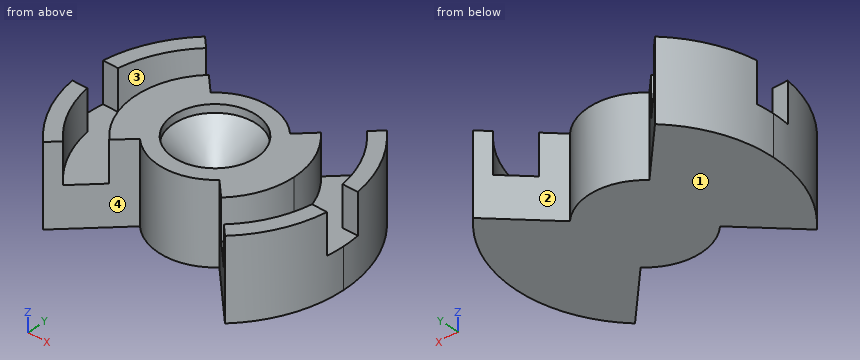
```python
from build123d import *

# Parameters (mm, degrees)
F0_R     = 3.27025
F1_DEPTH = 6.35
F2_R     = 3.27025
F3_DEPTH = 3.175
F4_SIZE  = 2.54


# Not quite as in the source:
# - a feature names something its author has since deleted; it is built from what else it names


with BuildPart() as f1:
    # F0 (on Top) → F1 (new body)
    with BuildSketch(Plane.XY):
        with BuildLine():
            ThreePointArc((-4.445, 0), (-4.106644522, 1.7010278569), (-3.1430896424, 3.1430896424))
            Line((-3.1430896424, 3.1430896424), (-7.1842048969, 7.1842048969))
            ThreePointArc((-7.1842048969, 7.1842048969), (-9.3866160503, 3.8880636728), (-10.16, 0))
            ThreePointArc((-10.16, 0), (-9.3866160503, -3.8880636728), (-7.1842048969, -7.1842048969))
            Line((-7.1842048969, -7.1842048969), (-3.1430896424, -3.1430896424))
            ThreePointArc((-3.1430896424, -3.1430896424), (-4.106644522, -1.7010278569), (-4.445, 0))
        make_face()
        with BuildLine():
            ThreePointArc((3.1430896424, -3.1430896424), (4.106644522, -1.7010278569), (4.445, 0))
            ThreePointArc((4.445, 0), (4.106644522, 1.7010278569), (3.1430896424, 3.1430896424))
            ThreePointArc((3.1430896424, 3.1430896424), (0, 4.445), (-3.1430896424, 3.1430896424))
            ThreePointArc((-3.1430896424, 3.1430896424), (-4.106644522, 1.7010278569), (-4.445, 0))
            ThreePointArc((-4.445, 0), (-4.106644522, -1.7010278569), (-3.1430896424, -3.1430896424))
            ThreePointArc((-3.1430896424, -3.1430896424), (0, -4.445), (3.1430896424, -3.1430896424))
        make_face()
        Circle(F0_R, mode=Mode.SUBTRACT)
        with BuildLine():
            ThreePointArc((3.1430896424, 3.1430896424), (4.106644522, 1.7010278569), (4.445, 0))
            ThreePointArc((4.445, 0), (4.106644522, -1.7010278569), (3.1430896424, -3.1430896424))
            Line((3.1430896424, -3.1430896424), (7.1842048969, -7.1842048969))
            ThreePointArc((7.1842048969, -7.1842048969), (9.3866160503, -3.8880636728), (10.16, 0))
            ThreePointArc((10.16, 0), (9.3866160503, 3.8880636728), (7.1842048969, 7.1842048969))
            Line((7.1842048969, 7.1842048969), (3.1430896424, 3.1430896424))
        make_face()
        Circle(F0_R)
    extrude(amount=F1_DEPTH)

    # F2 (on face) → F3 (cut)
    with BuildSketch(Plane.XY.offset(6.35)):
        with BuildLine():
            ThreePointArc((-4.4227761396, -4.4227761396), (-6.25475, 0), (-4.4227761396, 4.4227761396))
            Line((-4.4227761396, 4.4227761396), (-6.3535312057, 6.3535312057))
            ThreePointArc((-6.3535312057, 6.3535312057), (-8.0151664506, 4.0610127224), (-8.8809239384, 1.36525))
            ThreePointArc((-8.8809239384, 1.36525), (-8.98525, 0), (-8.8809239384, -1.36525))
            ThreePointArc((-8.8809239384, -1.36525), (-8.0151664506, -4.0610127224), (-6.3535312057, -6.3535312057))
            Line((-6.3535312057, -6.3535312057), (-4.4227761396, -4.4227761396))
        make_face()
        with BuildLine():
            ThreePointArc((4.4227761396, 4.4227761396), (5.778635506, 2.3935891986), (6.25475, 0))
            ThreePointArc((6.25475, 0), (5.778635506, -2.3935891986), (4.4227761396, -4.4227761396))
            Line((4.4227761396, -4.4227761396), (6.3535312057, -6.3535312057))
            ThreePointArc((6.3535312057, -6.3535312057), (8.0151664506, -4.0610127224), (8.8809239384, -1.36525))
            ThreePointArc((8.8809239384, -1.36525), (8.9591305209, -0.6846151272), (8.98525, 0))
            ThreePointArc((8.98525, 0), (8.9591305209, 0.6846151272), (8.8809239384, 1.36525))
            ThreePointArc((8.8809239384, 1.36525), (8.0151664506, 4.0610127224), (6.3535312057, 6.3535312057))
            Line((6.3535312057, 6.3535312057), (4.4227761396, 4.4227761396))
        make_face()
        with BuildLine():
            ThreePointArc((-8.8809239384, -1.36525), (-8.98525, 0), (-8.8809239384, 1.36525))
            Line((-8.8809239384, 1.36525), (-10.0678544108, 1.36525))
            ThreePointArc((-10.0678544108, 1.36525), (-10.16, 0), (-10.0678544108, -1.36525))
            Line((-10.0678544108, -1.36525), (-8.8809239384, -1.36525))
        make_face()
        with BuildLine():
            Line((10.0678544108, 1.36525), (8.8809239384, 1.36525))
            ThreePointArc((8.8809239384, 1.36525), (8.9591305209, 0.6846151272), (8.98525, 0))
            ThreePointArc((8.98525, 0), (8.9591305209, -0.6846151272), (8.8809239384, -1.36525))
            Line((8.8809239384, -1.36525), (10.0678544108, -1.36525))
            ThreePointArc((10.0678544108, -1.36525), (10.16, 0), (10.0678544108, 1.36525))
        make_face()
        Circle(F2_R)
    extrude(amount=-F3_DEPTH, mode=Mode.SUBTRACT)

    # F4
    f4_edges = [f1.edges().sort_by_distance(p)[0] for p in [
        (-3.27025, 0, 3.175),
    ]]
    chamfer(f4_edges, length=F4_SIZE)


solid = f1.part
```
Part model, mm, in its own coordinate system. Face numbers are marked on the shaded views. A direction names the side the tool comes from. Give positions to 0.01 mm unless a question says otherwise; leave off trailing zeros. Write each loop counter-clockwise with the first axis right and the second up, starting at its lowest first coordinate (ties: lowest second). Pieces come first, ordered by that corner, then holes. Notation, with made-up numbers: (-35, 2.25) -> (-25, 2.25) arc R23 cw to (-25, 18.25) -> close; hole circle Ø6 at (72.25, 36.25). An arc over 180 degrees is marked (long way). Put each result on its own line as item: value. Start each with the question number.
Item 1: Cut at C-C (x = 0). List the corners of the cut face in (y, z) (3 decimals).
Item 2: Pin check, flat tips, straight feed: pin 1 Ø1.7 at (x, y) = (-8, -0.5) entering from +Z (3 decimals); pin 2 Ø3 at (y, z) = (-1, 3.5) entering from +X; pin 3 Ø1.2 at (x, y) = (0, 0.5) entering from +Z; pin 4 Ø1.3 at (x, z) = (-9.5, 4) entering from +Y. Stop position of each tip, or through.
Item 3: Cut at B-B (y = -5). List the corners of the cut face in (x, z) (3 decimals), then the cut area to 3 significant figures.
Item 4: Which spindle directions (+Z, -Z, +X, -X, +Y, -Y) get a long thin tool onto all of the face, cutting with end or side? Do the marked faces 1, 2, 3 and 4. Say none if no direction does.
Item 5: Cut at D-D (z = 1). List the corners of the cut face in (x, y) (3 decimals).
Item 6: Wall check: L1, parallel to Y at x = 0, z = 6.15 (3 decimals); L2, parallel to Z at x = -7, y = -5.5 (3 decimals); L3, parallel to X at y = -4, z = 3.5. Give the ranges that are in metal, low to high. Write a range as [from, to].
Item 7: Cut at A-A (z = 3.5). List the corners of the cut face in (x, y) (1 decimal).
Answer list:
1. outline: (-4.445, 0) -> (4.445, 0) -> (4.445, 6.35) -> (3.27, 6.35) -> (3.27, 5.715) -> (0.73, 3.175) -> (-0.73, 3.175) -> (-3.27, 5.715) -> (-3.27, 6.35) -> (-4.445, 6.35) -> close
2. pin 1: stops at z = 3.175
2. pin 2: stops at x = 10.16
2. pin 3: stops at z = 3.54
2. pin 4: stops at y = 4.99
3. outline: (-8.845, 0) -> (-5, 0) -> (-5, 3.175) -> (-7.466, 3.175) -> (-7.466, 6.35) -> (-8.845, 6.35) -> close; (5, 0) -> (8.845, 0) -> (8.845, 6.35) -> (7.466, 6.35) -> (7.466, 3.175) -> (5, 3.175) -> close
3. area: 33.2 mm2
4. face 1: -Z, +X, -X, +Y, -Y
4. face 2: +Z, -Z, +Y
4. face 3: +Z
4. face 4: +Z, -Z, -Y
5. outline: (-7.184, -7.184) -> (-3.143, -3.143) arc R4.445 ccw to (3.143, -3.143) -> (7.184, -7.184) arc R10.16 ccw to (7.184, 7.184) -> (3.143, 3.143) arc R4.445 ccw to (-3.143, 3.143) -> (-7.184, 7.184) arc R10.16 ccw to start
6. L1: y = [-4.445, -3.27], [3.27, 4.445]
6. L2: z = [0, 3.175]
6. L3: x = [-9.34, -8.05], [-4.81, -4], [-1.94, 1.94], [4, 4.81], [8.05, 9.34]
7. outline: (-10.1, -1.4) arc R10.2 ccw to (-7.2, -7.2) -> (-6.4, -6.4) arc R9 cw to (-8.9, -1.4) -> close; (-10.1, 1.4) -> (-8.9, 1.4) arc R9 cw to (-6.4, 6.4) -> (-7.2, 7.2) arc R10.2 ccw to start; (-4.4, -4.4) -> (-3.1, -3.1) arc R4.4 ccw to (3.1, -3.1) -> (4.4, -4.4) arc R6.3 ccw to (4.4, 4.4) -> (3.1, 3.1) arc R4.4 ccw to (-3.1, 3.1) -> (-4.4, 4.4) arc R6.3 ccw to start; (6.4, -6.4) -> (7.2, -7.2) arc R10.2 ccw to (10.1, -1.4) -> (8.9, -1.4) arc R9 cw to start; (6.4, 6.4) arc R9 cw to (8.9, 1.4) -> (10.1, 1.4) arc R10.2 ccw to (7.2, 7.2) -> close; hole circle Ø2.1 at (0, 0)
